Verification items for the finished model (mm, model axes). A direction names the side the tool comes from. Give positions to 0.01 mm unless a question says otherwise; leave off trailing zeros. Loops run counter-clockwise (first coordinate to the right, second up) from the corner with the lowest first, then second, coordinate; pieces in that order, holes last. Notation, with made-up numbers: (71.25, -38.75) -> (76.25, -38.75) arc R34 cw to (76.25, -4.75) -> close; hole circle Ø8 at (-5, 71.25). An arc over 180 degrees is marked (long way). Answer in a Markdown table with one row per item. Add a question column.
Q1. Material ranges on probe 1 along X at (y, z) = (2.5, -21.25); probe 2 along X at (y, z) = (-0.75, -13.75); probe 3 along Y at (x, z) = (-3, -23), recorded low to high.
Q2. Section check A-A on x = -9.25. Enter the section's corners in (y, z), and give its area (3 significant figures).
Q3. Release check for a two-part mould opening along Y. For faces 1 (the face through (-12, 3, -13)), 2 (the face through (0, -1, -23.707)), 3 (the face through (10, 5, -24)), 4 (the face through (12.79, 4.98, -6.11)) record: pulls with the +Y half, pulls with the -Y half, needs draft (parallel to the pull), parting line crosses it, or undercut.
Q4. Gauge pin test, flat ends, axial feed: P1, Ø6.5, axis at y = 4.83, z = -11.21, coming from the +X side; P2, Ø1, axis at y = 4.5, z = -24.5, coming from the -X side; P3, Ø1.3, axis at x = 4, y = -0.5, coming from the -Z side; P4, Ø3.5, axis at y = 4.83, z = -11.21, coming from the -X side. Record the tip position at first contact, or that the pin passes through.
Q5. Section check D-D on z = -17. Enter the section's corners in (x, y), and give its area (3 significant figures).
Q6. Section check B-B on y = 9.5. Enter the section's corners in (x, z).
Q7. Set-up check for faces 5 (the face through (-13.2, 4.8, -24.5)), 6 (the face through (11, 5, -17.977)), 7 (the face through (-11.6, 6, -24)): record each of +Z, -Z, +X, -X, +Y, -Y from which the full face is reachable in a straight line by a thin tool's end or side.
Q8. Section check C-C on z = -28.25. Enter the section's corners in (x, y), and give its area (3 significant figures).
```python
from build123d import *

# Parameters (mm, degrees)
F2_DEPTH = 1.6
F3_DEPTH = 2
F4_DEPTH = 0.4
F5_DEPTH = 11.6
F6_DEPTH = 2
F7_DEPTH = 1.6
F9_DEPTH = 25


# Not quite as in the source:
# - a feature names something its author has since deleted; it is built from what else it names


with BuildPart() as f2:
    # F1 (on offset) → F2 (new body)
    with BuildSketch(Plane.YZ.offset(11.6)):
        with BuildLine():
            Line((-0.1658547654, -17.9765316878), (-0.1658547654, -20.645576419))
            ThreePointArc((-0.1658547654, -20.645576419), (4.8341452346, -18.4390658066), (9.8341452346, -20.645576419))
            Line((9.8341452346, -20.645576419), (9.8341452346, -17.9765316878))
            Line((9.8341452346, -17.9765316878), (-0.1658547654, -17.9765316878))
        make_face()
        with BuildLine():
            Line((-0.1658547654, -23.7073743102), (-1.7658547654, -23.7073743102))
            Line((-1.7658547654, -23.7073743102), (-1.7658547654, -25.2073743102))
            Line((-1.7658547654, -25.2073743102), (-0.1658547654, -25.2073743102))
            Line((-0.1658547654, -25.2073743102), (3.1570942515, -25.2073743102))
            ThreePointArc((3.1570942515, -25.2073743102), (4.8341452346, -23.9573743102), (6.5111962178, -25.2073743102))
            Line((6.5111962178, -25.2073743102), (9.8341452346, -25.2073743102))
            Line((9.8341452346, -25.2073743102), (11.4341452346, -25.2073743102))
            Line((11.4341452346, -25.2073743102), (11.4341452346, -23.7073743102))
            Line((11.4341452346, -23.7073743102), (9.8341452346, -23.7073743102))
            Line((9.8341452346, -23.7073743102), (9.8341452346, -20.645576419))
            ThreePointArc((9.8341452346, -20.645576419), (4.8341452346, -18.4390658066), (-0.1658547654, -20.645576419))
            Line((-0.1658547654, -20.645576419), (-0.1658547654, -23.7073743102))
        make_face()
        with BuildLine():
            Line((-0.1658547654, -25.2073743102), (-1.7658547654, -25.2073743102))
            ThreePointArc((-1.7658547654, -25.2073743102), (-0.9246460766, -28.0854161792), (1.3341452346, -30.0573743102))
            Line((1.3341452346, -30.0573743102), (8.3341452346, -30.0573743102))
            ThreePointArc((8.3341452346, -30.0573743102), (10.5929365459, -28.0854161792), (11.4341452346, -25.2073743102))
            Line((11.4341452346, -25.2073743102), (9.8341452346, -25.2073743102))
            Line((9.8341452346, -25.2073743102), (6.5111962178, -25.2073743102))
            ThreePointArc((6.5111962178, -25.2073743102), (6.5658119492, -25.4547275414), (6.5841452346, -25.7073743102))
            ThreePointArc((6.5841452346, -25.7073743102), (4.5814984659, -27.4390410247), (3.1570942515, -25.2073743102))
            Line((3.1570942515, -25.2073743102), (-0.1658547654, -25.2073743102))
        make_face()
        with BuildLine():
            Line((6.5111962178, -25.2073743102), (3.1570942515, -25.2073743102))
            ThreePointArc((3.1570942515, -25.2073743102), (4.5814984659, -27.4390410247), (6.5841452346, -25.7073743102))
            ThreePointArc((6.5841452346, -25.7073743102), (6.5658119492, -25.4547275414), (6.5111962178, -25.2073743102))
        make_face()
        with BuildLine():
            ThreePointArc((6.5111962178, -25.2073743102), (4.8341452346, -23.9573743102), (3.1570942515, -25.2073743102))
            Line((3.1570942515, -25.2073743102), (6.5111962178, -25.2073743102))
        make_face()
        with BuildLine():
            Line((9.8341452346, -23.7073743102), (11.4341452346, -23.7073743102))
            ThreePointArc((11.4341452346, -23.7073743102), (10.8327827117, -22.0726736198), (9.8341452346, -20.645576419))
            Line((9.8341452346, -20.645576419), (9.8341452346, -23.7073743102))
        make_face()
        with BuildLine():
            ThreePointArc((-0.1658547654, -20.645576419), (-1.1644922425, -22.0726736198), (-1.7658547654, -23.7073743102))
            Line((-1.7658547654, -23.7073743102), (-0.1658547654, -23.7073743102))
            Line((-0.1658547654, -23.7073743102), (-0.1658547654, -20.645576419))
        make_face()
    extrude(amount=-F2_DEPTH)

    # F1 (on offset) → F3 (join)
    with BuildSketch(Plane.YZ.offset(11.6)):
        with BuildLine():
            Line((-0.1658547654, -12.7073743102), (-1.7658547654, -12.7073743102))
            Line((-1.7658547654, -12.7073743102), (-1.7658547654, -14.7073743102))
            Line((-1.7658547654, -14.7073743102), (-0.1658547654, -14.7073743102))
            Line((-0.1658547654, -14.7073743102), (-0.1658547654, -17.9765316878))
            Line((-0.1658547654, -17.9765316878), (9.8341452346, -17.9765316878))
            Line((9.8341452346, -17.9765316878), (9.8341452346, -14.7278557842))
            Line((9.8341452346, -14.7278557842), (11.4341452346, -14.7073743102))
            Line((11.4341452346, -14.7073743102), (11.4341452346, -12.7073743102))
            Line((11.4341452346, -12.7073743102), (9.8341452346, -12.7073743102))
            Line((9.8341452346, -12.7073743102), (6.1570208902, -12.7073743102))
            ThreePointArc((6.1570208902, -12.7073743102), (4.8341452346, -13.2073743102), (3.5112695791, -12.7073743102))
            Line((3.5112695791, -12.7073743102), (-0.1658547654, -12.7073743102))
        make_face()
        with BuildLine():
            ThreePointArc((11.4341452346, -12.7073743102), (4.8341452346, -6.1073743102), (-1.7658547654, -12.7073743102))
            Line((-1.7658547654, -12.7073743102), (-0.1658547654, -12.7073743102))
            Line((-0.1658547654, -12.7073743102), (3.5112695791, -12.7073743102))
            ThreePointArc((3.5112695791, -12.7073743102), (4.0112695791, -9.3844986547), (6.8341452346, -11.2073743102))
            ThreePointArc((6.8341452346, -11.2073743102), (6.6570208902, -12.0302499657), (6.1570208902, -12.7073743102))
            Line((6.1570208902, -12.7073743102), (9.8341452346, -12.7073743102))
            Line((9.8341452346, -12.7073743102), (11.4341452346, -12.7073743102))
        make_face()
        with BuildLine():
            Line((-0.1658547654, -17.9765316878), (-0.1658547654, -20.645576419))
            ThreePointArc((-0.1658547654, -20.645576419), (4.8341452346, -18.4390658066), (9.8341452346, -20.645576419))
            Line((9.8341452346, -20.645576419), (9.8341452346, -17.9765316878))
            Line((9.8341452346, -17.9765316878), (-0.1658547654, -17.9765316878))
        make_face()
    extrude(amount=F3_DEPTH)

    # F1 (on offset) → F4 (cut)
    with BuildSketch(Plane.YZ.offset(11.6)):
        with BuildLine():
            Line((-0.1658547654, -12.7073743102), (-1.7658547654, -12.7073743102))
            Line((-1.7658547654, -12.7073743102), (-1.7658547654, -14.7073743102))
            Line((-1.7658547654, -14.7073743102), (-0.1658547654, -14.7073743102))
            Line((-0.1658547654, -14.7073743102), (-0.1658547654, -17.9765316878))
            Line((-0.1658547654, -17.9765316878), (9.8341452346, -17.9765316878))
            Line((9.8341452346, -17.9765316878), (9.8341452346, -14.7278557842))
            Line((9.8341452346, -14.7278557842), (11.4341452346, -14.7073743102))
            Line((11.4341452346, -14.7073743102), (11.4341452346, -12.7073743102))
            Line((11.4341452346, -12.7073743102), (9.8341452346, -12.7073743102))
            Line((9.8341452346, -12.7073743102), (6.1570208902, -12.7073743102))
            ThreePointArc((6.1570208902, -12.7073743102), (4.8341452346, -13.2073743102), (3.5112695791, -12.7073743102))
            Line((3.5112695791, -12.7073743102), (-0.1658547654, -12.7073743102))
        make_face()
        with BuildLine():
            ThreePointArc((11.4341452346, -12.7073743102), (4.8341452346, -6.1073743102), (-1.7658547654, -12.7073743102))
            Line((-1.7658547654, -12.7073743102), (-0.1658547654, -12.7073743102))
            Line((-0.1658547654, -12.7073743102), (3.5112695791, -12.7073743102))
            ThreePointArc((3.5112695791, -12.7073743102), (4.0112695791, -9.3844986547), (6.8341452346, -11.2073743102))
            ThreePointArc((6.8341452346, -11.2073743102), (6.6570208902, -12.0302499657), (6.1570208902, -12.7073743102))
            Line((6.1570208902, -12.7073743102), (9.8341452346, -12.7073743102))
            Line((9.8341452346, -12.7073743102), (11.4341452346, -12.7073743102))
        make_face()
    extrude(amount=F4_DEPTH, mode=Mode.SUBTRACT)



with BuildPart() as f5:
    # F1 (on offset) → F5 (new body)
    with BuildSketch(Plane.YZ.offset(11.6)):
        with BuildLine():
            Line((11.4341452346, -23.7073743102), (11.4341452346, -14.7073743102))
            Line((11.4341452346, -14.7073743102), (9.8341452346, -14.7278557842))
            Line((9.8341452346, -14.7278557842), (9.8341452346, -17.9765316878))
            Line((9.8341452346, -17.9765316878), (9.8341452346, -20.645576419))
            ThreePointArc((9.8341452346, -20.645576419), (10.8327827117, -22.0726736198), (11.4341452346, -23.7073743102))
        make_face()
        with BuildLine():
            Line((9.8341452346, -23.7073743102), (11.4341452346, -23.7073743102))
            ThreePointArc((11.4341452346, -23.7073743102), (10.8327827117, -22.0726736198), (9.8341452346, -20.645576419))
            Line((9.8341452346, -20.645576419), (9.8341452346, -23.7073743102))
        make_face()
    extrude(amount=-F5_DEPTH)


with BuildPart() as f5b:
    # F1 (on offset) → F5, piece 2 (new body)
    with BuildSketch(Plane.YZ.offset(11.6)):
        with BuildLine():
            Line((-0.1658547654, -14.7073743102), (-1.7658547654, -14.7073743102))
            Line((-1.7658547654, -14.7073743102), (-1.7658547654, -23.7073743102))
            ThreePointArc((-1.7658547654, -23.7073743102), (-1.1644922425, -22.0726736198), (-0.1658547654, -20.645576419))
            Line((-0.1658547654, -20.645576419), (-0.1658547654, -17.9765316878))
            Line((-0.1658547654, -17.9765316878), (-0.1658547654, -14.7073743102))
        make_face()
        with BuildLine():
            ThreePointArc((-0.1658547654, -20.645576419), (-1.1644922425, -22.0726736198), (-1.7658547654, -23.7073743102))
            Line((-1.7658547654, -23.7073743102), (-0.1658547654, -23.7073743102))
            Line((-0.1658547654, -23.7073743102), (-0.1658547654, -20.645576419))
        make_face()
    extrude(amount=-F5_DEPTH)


with BuildPart() as f2_1:
    add(f2.part)

    add(f5.part)  # F6 merges F5

    add(f5b.part)  # F6 merges F5b
    # F1 (on offset) → F6 (join)
    with BuildSketch(Plane.YZ.offset(11.6)):
        with BuildLine():
            Line((-0.1658547654, -14.7073743102), (-1.7658547654, -14.7073743102))
            Line((-1.7658547654, -14.7073743102), (-1.7658547654, -23.7073743102))
            ThreePointArc((-1.7658547654, -23.7073743102), (-1.1644922425, -22.0726736198), (-0.1658547654, -20.645576419))
            Line((-0.1658547654, -20.645576419), (-0.1658547654, -17.9765316878))
            Line((-0.1658547654, -17.9765316878), (-0.1658547654, -14.7073743102))
        make_face()
        with BuildLine():
            Line((11.4341452346, -23.7073743102), (11.4341452346, -14.7073743102))
            Line((11.4341452346, -14.7073743102), (9.8341452346, -14.7278557842))
            Line((9.8341452346, -14.7278557842), (9.8341452346, -17.9765316878))
            Line((9.8341452346, -17.9765316878), (9.8341452346, -20.645576419))
            ThreePointArc((9.8341452346, -20.645576419), (10.8327827117, -22.0726736198), (11.4341452346, -23.7073743102))
        make_face()
    extrude(amount=F6_DEPTH)

    # F1 (on offset) → F7 (join)
    with BuildSketch(Plane.YZ.offset(11.6)):
        with BuildLine():
            ThreePointArc((6.5111962178, -25.2073743102), (4.8341452346, -23.9573743102), (3.1570942515, -25.2073743102))
            Line((3.1570942515, -25.2073743102), (6.5111962178, -25.2073743102))
        make_face()
        with BuildLine():
            Line((6.5111962178, -25.2073743102), (3.1570942515, -25.2073743102))
            ThreePointArc((3.1570942515, -25.2073743102), (4.5814984659, -27.4390410247), (6.5841452346, -25.7073743102))
            ThreePointArc((6.5841452346, -25.7073743102), (6.5658119492, -25.4547275414), (6.5111962178, -25.2073743102))
        make_face()
    extrude(amount=F7_DEPTH)

    # F8 (on Front) → F9 (cut)
    with BuildSketch(Plane.XZ):
        Polygon((14.5103234728, -25.0094107672), (13.301373871, -24.5876735715), (12.2712288238, -27.5406818837), (13.4801784256, -27.9624190794), align=None)
    extrude(amount=-F9_DEPTH, mode=Mode.SUBTRACT)

    # F10: F2 across plane


with BuildPart() as f2_2:
    add(f2_1.part)
    add(f2_1.part.mirror(Plane.YZ))


with BuildPart() as f11_1:
    # F11: copy of F2
    add(f2_2.part)


solid = f2_2.part
```
Taken from the geometry:
| question | item | result |
|---|---|---|
| 1 | probe 1 | x = -11.6 to -10, 10 to 11.6 |
| 1 | probe 2 | x = -13.6 to -12, 12 to 13.6 |
| 1 | probe 3 | y = -1.77 to -0.17, 9.83 to 11.43 |
| 2 | outline | (-1.77, -23.71) -> (-0.17, -23.71) -> (-0.17, -14.71) -> (-1.77, -14.71) -> close; (9.83, -23.71) -> (11.43, -23.71) -> (11.43, -14.71) -> (9.83, -14.73) -> close |
| 2 | area | 28.8 mm² |
| 3 | face 1 | undercut |
| 3 | face 2 | needs draft |
| 3 | face 3 | undercut |
| 3 | face 4 | parting line crosses it |
| 4 | P1 | stops at x = 13.6 |
| 4 | P2 | stops at x = -13.2 |
| 4 | P3 | stops at z = -23.71 |
| 4 | P4 | passes through |
| 5 | outline | (-13.6, -1.77) -> (13.6, -1.77) -> (13.6, 11.43) -> (-13.6, 11.43) -> close; hole (-12, -0.17) -> (12, -0.17) -> (12, 9.83) -> (-12, 9.83) -> close |
| 5 | area | 119 mm² |
| 6 | outline | (-13.6, -20.3) -> (-11.6, -20.3) -> (-11.6, -29.32) -> (-10, -29.32) -> (-10, -17.98) -> (-12, -17.98) -> (-12, -8.04) -> (-13.6, -8.04) -> close; (10, -29.32) -> (11.6, -29.32) -> (11.6, -20.3) -> (13.6, -20.3) -> (13.6, -8.04) -> (12, -8.04) -> (12, -17.98) -> (10, -17.98) -> close |
| 7 | face 5 | -Z, -X, +Y, -Y |
| 7 | face 6 | +Z |
| 7 | face 7 | -X |
| 8 | outline | (-11.6, -0.82) -> (-10, -0.82) -> (-10, 10.48) -> (-11.6, 10.48) -> close; (10, -0.82) -> (11.6, -0.82) -> (11.6, 10.48) -> (10, 10.48) -> close |
| 8 | area | 36.2 mm² |
